Verification items for the finished model (mm, model axes). A direction names the side the tool comes from. Coordinates: 2 decimals unless noted, no trailing zeros. Order: outer loops, then holes, each group sorted by start corner. A loop starts at its lowest first (then second) coordinate and runs counter-clockwise, first axis right, second up. Notation, with made-up numbers: M 13,39.5 L 28,39.5 A17 cw 28,44.5 Z; hole C 8,-6.5 d8. An arc over 180 degrees is marked long. Return JSON: item names as keys, results as strings. Group by question number.
1. Set-up check for faces 4 (the flat face through (60, 2, 42.875)), 5 (the flat face through (22.225, -17, 18)), 6 (the cylindrical face through (32.112, 16.547, 51.348)), 7 (the flat face through (46, -25.4, 42)), 8 (the flat face through (46, 25.4, 42)): record each of +Z, -Z, +X, -X, +Y, -Y from which the full face is reachable in a straight line by a thin tool's end or side.
2. Mould release check, pull along X, two halves, no side actions. Record for faces 1 (the cylindrical face through (45.8, -0.4, 38.1)), 2 (the flat face through (-3, 7.938, 30)), 3 (the flat face through (-41.275, -1, 0)): +X half, -X half, draft (parallel to the pull), parting line (faces both ways), or undercut.
3. Material ranges on line 1 along X through (y, z) = (-7.5, 1) (3 decimals); line 2 along Y through (x, z) = (5.5, 49); line 3 along Y through (x, z) = (61, 49), recorded low to high.
4. Gauge pin test, flat ends, axial feed: pin 1 (19 mm diameter, centred on y = -18, z = 18, fed in from -X) (3 decimals); pin 2 (15.5 mm diameter, centred on x = -2, z = 42, fed in from -Y); pin 3 (14.5 mm diameter, centred on x = 69, y = 9.5, fed in from -Z); pin 4 (1 mm diameter, centred on y = 15.5, z = 54.5, fed in from +X). Record the tip position at first contact, or that the pin passes through.
5. Section check A-A, the plane y = 30. Record the cut outline in (x, z) (3 decimals).
```python
from build123d import *

# Parameters (mm, degrees)
F1_DEPTH = 63.5
F0_W     = 25.4
F0_H     = 19.05
F2_DEPTH = 25.4
F3_DEPTH = 7.9375
F5_R     = 5.08


# Not quite as in the source:
# - ends of sketch curves that miss each other by under 0.0002 mm in the source are joined


with BuildPart() as f1:
    # F0 (on Front) → F1 (new body, symmetric)
    with BuildSketch(Plane.XZ):
        Polygon((-41.275, -9.525), (41.275, -9.525), (41.275, 9.525), (22.225, 9.525), (-41.275, 9.525), align=None)
    extrude(amount=F1_DEPTH, both=True)

    # F0 (on Front) → F2 (join, symmetric)
    with BuildSketch(Plane.XZ):
        with BuildLine():
            Line((22.225, 9.525), (41.275, 9.525))
            Line((41.275, 9.525), (41.275, 27.0002))
            ThreePointArc((41.275, 27.0002), (45.9246798487, 38.2255201513), (57.15, 42.8752))
            Line((57.15, 42.8752), (60.325, 42.8752))
            Line((60.325, 42.8752), (60.325, 61.9252))
            Line((60.325, 61.9252), (57.15, 61.9252))
            add(Edge.make_bspline(
                [(55.4308013552, 61.8828601769), (56.0086976587, 61.9022725241), (56.5818561966, 61.916408872), (57.15, 61.9252)],
                knots=[109.8295826069, 109.8295826069, 109.8295826069, 109.8295826069, 111.5045361635, 111.5045361635, 111.5045361635, 111.5045361635], degree=3))
            ThreePointArc((55.4308013552, 61.8828601769), (31.8537686832, 51.0804056919), (22.225, 27.0002))
            Line((22.225, 27.0002), (22.225, 9.525))
        make_face()
        with Locations((73.025, 52.4002)):
            Rectangle(F0_W, F0_H)
    extrude(amount=F2_DEPTH, both=True)

    # F0 (on Front) → F3 (join, symmetric)
    with BuildSketch(Plane.XZ):
        with BuildLine():
            add(Edge.make_bspline(
                [(-41.275, 9.525), (-40.7272405937, 36.6521064094), (17.5371477958, 60.609959217), (55.4308013552, 61.8828601769)],
                knots=[0, 0, 0, 0, 109.8295826069, 109.8295826069, 109.8295826069, 109.8295826069], degree=3))
            Line((-41.275, 9.525), (22.225, 9.525))
            Line((22.225, 9.525), (22.225, 27.0002))
            ThreePointArc((22.225, 27.0002), (31.8537686832, 51.0804056919), (55.4308013552, 61.8828601769))
        make_face()
    extrude(amount=F3_DEPTH, both=True)

    # F0 (on Front) → F4 (revolve)
    with BuildSketch(Plane.XZ):
        Polygon((85.725, 61.9252), (85.725, 42.8752), (85.725, 38.1), (111.125, 38.1), (111.125, 66.675), (85.725, 66.675), align=None)
    revolve(axis=Axis((85.725, 0, 52.3875), (0, 0, -1)))

    # F5
    f5_edges = [f1.edges().sort_by_distance(p)[0] for p in [
        (41.275, -63.5, 0),
        (-41.275, -63.5, 0),
        (-41.275, 63.5, 0),
        (41.275, 63.5, 0),
    ]]
    fillet(f5_edges, radius=F5_R)


solid = f1.part
```
Answers follow:
{
 "1": {"face 4": "-Z", "face 5": "+Z, -X, -Y", "face 6": "+Z, -X, +Y", "face 7": "+Z, +X, -X, -Y", "face 8": "+Z, +X, -X, +Y"},
 "2": {"face 1": "undercut", "face 2": "draft", "face 3": "-X half"},
 "3": {"line 1": "-41.275 to 41.275", "line 2": "-7.94 to 7.94", "line 3": "-25.4 to 25.4"},
 "4": {"pin 1": "x = -41.275", "pin 2": "y = -7.94", "pin 3": "z = 38.1", "pin 4": "x = 106.22"},
 "5": {"outline": "M -41.275,-9.525 L 41.275,-9.525 L 41.275,9.525 L -41.275,9.525 Z"}
}
